```python
from build123d import *

# Parameters (mm, degrees)
SZKIC1_R                    = 81
SZKIC1_R_2                  = 75
DODANIE_WYCI_GNI_CIE1_DEPTH = 2
SZKIC2_R                    = 1.5
WYTNIJ_WYCI_GNI_CIE1_DEPTH  = 2
SZYK_KO_OWY1_COUNT          = 8


with BuildPart() as part:
    # Szkic1 → Dodanie-wyciągnięcie1 (new body)
    with BuildSketch(Plane.XY):
        Circle(SZKIC1_R)
        Circle(SZKIC1_R_2, mode=Mode.SUBTRACT)
    extrude(amount=DODANIE_WYCI_GNI_CIE1_DEPTH)

    # Szkic2 → Wytnij-wyciągnięcie1 (cut)
    with BuildSketch(Plane.XY.offset(2)):
        with Locations((0, 78)):
            Circle(SZKIC2_R)
    wytnij_wyci_gni_cie1 = extrude(amount=-WYTNIJ_WYCI_GNI_CIE1_DEPTH, mode=Mode.SUBTRACT)

    # Szyk kołowy1: Wytnij-wyciągnięcie1 ×8 about axis
    szyk_ko_owy1_axis = Axis((0, 0, 0), (0, 0, 1))
    for i in range(1, SZYK_KO_OWY1_COUNT):
        add(wytnij_wyci_gni_cie1.rotate(szyk_ko_owy1_axis, i * 360 / SZYK_KO_OWY1_COUNT), mode=Mode.SUBTRACT)


solid = part.part
```
Work out the finished part from the listing and answer in its coordinate system (mm). Round coordinates to 2 decimals unless told otherwise and drop trailing zeros. Write each loop counter-clockwise with the first axis right and the second up, starting at its lowest first coordinate (ties: lowest second). Pieces come first, ordered by that corner, then holes. Notation, with made-up numbers: (75, -3.5) - (115, -3.5) arc R28 ccw to (115, 31.5) - close; hole circle Ø1 at (70, 68.25). An arc over 180 degrees is marked (long way). Return JSON: item names as keys, results as strings. Group by question number.
Q1. Each of these flat-tipped pins is pushed along its axis until it touches: pin 1 Ø2.5 at (x, y) = (0, 78) entering from +Z; pin 2 Ø1 at (x, z) = (40, 1) entering from -Y; pin 3 Ø1 at (y, z) = (51.5, 1) entering from +X. Where does it stop, or does it pass through?
Q2. Find the intervals of material crossed by L1, parallel to Y at x = 0, z = 1.1; L2, parallel to Y at x = 54, z = 0.4; L3, parallel to X at y = 1, z = 1.4, in increasing order.
Q3. The mould has two halves that part along X. Classify faces 1 (the cylindrical face through (-9.764, 74.362, 0.986)), 2 (the flat face through (72, -24, 2)), 3 (the cylindrical face through (43.545, 68.3, 0.986)): released by +X, released by -X, zero draft, split by the parting line, or undercut.
Q4. The part is cut by section C-C on z = 1.1. Count the separate pieces of the cut face and the enclosed holes in it, then the cut area to 3 significant figures.
Q5. The part is cut by section B-B on x = -12.5. Write down the section's boundary in (y, z), then the cut area to 3 significant figures.
Q6. The part is cut by section A-A on y = 62. Write down the section's boundary in (x, z).
Solved:
{
 "1": {"pin 1": "through", "pin 2": "y = -70.72", "pin 3": "x = 62.93"},
 "2": {"L1": "-81 to -79.5, -76.5 to -75, 75 to 76.5, 79.5 to 81", "L2": "-60.37 to -56.11, -54.2 to -52.05, 52.05 to 54.2, 56.11 to 60.37", "L3": "-80.99 to -79.12, -76.88 to -74.99, 74.99 to 76.88, 79.12 to 80.99"},
 "3": {"face 1": "undercut", "face 2": "zero draft", "face 3": "split by the parting line"},
 "4": {"separate pieces": "1", "enclosed holes": "9", "area": "2,880 mm²"},
 "5": {"outline": "(-80.03, 0) - (-73.95, 0) - (-73.95, 2) - (-80.03, 2) - close; (73.95, 0) - (80.03, 0) - (80.03, 2) - (73.95, 2) - close", "area": "24.3 mm²"},
 "6": {"outline": "(-52.12, 0) - (-42.2, 0) - (-42.2, 2) - (-52.12, 2) - close; (42.2, 0) - (52.12, 0) - (52.12, 2) - (42.2, 2) - close"}
}
